from build123d import *

# Parameters (mm, degrees)
BOSS_EXTRUDE1_DEPTH   = 1.6
SKETCH2_R             = 3.45
BOSS_EXTRUDE2_DEPTH   = 1.4
M3X0_5_TAPPED_HOLE1_D = 2.5


with BuildPart() as part:
    # Sketch1 → Boss-Extrude1 (new body)
    with BuildSketch(Plane.XY):
        with BuildLine():
            Line((-6.237396753, 4.481095129), (-3, 5))
            Line((-3, 5), (3, 5))
            Line((3, 5), (6.237396753, 4.481095129))
            ThreePointArc((6.237396753, 4.481095129), (7.141511088, 3.973114811), (7.5, 3))
            Line((7.5, 3), (7.5, -3))
            ThreePointArc((7.5, -3), (7.141511088, -3.973114811), (6.237396753, -4.481095129))
            Line((6.237396753, -4.481095129), (3, -5))
            Line((3, -5), (-3, -5))
            Line((-3, -5), (-6.237396753, -4.481095129))
            ThreePointArc((-6.237396753, -4.481095129), (-7.141511088, -3.973114811), (-7.5, -3))
            Line((-7.5, -3), (-7.5, 3))
            ThreePointArc((-7.5, 3), (-7.141511088, 3.973114811), (-6.237396753, 4.481095129))
        make_face()
    extrude(amount=BOSS_EXTRUDE1_DEPTH)

    # Sketch2 → Boss-Extrude2 (add)
    with BuildSketch(Plane.XY.offset(1.6)):
        Circle(SKETCH2_R)
    extrude(amount=BOSS_EXTRUDE2_DEPTH)

    # M3x0.5 Tapped Hole1 (through all)
    with Locations(Plane.XY.offset(3)):
        with Locations((0, 0)):
            Hole(M3X0_5_TAPPED_HOLE1_D / 2)


solid = part.part
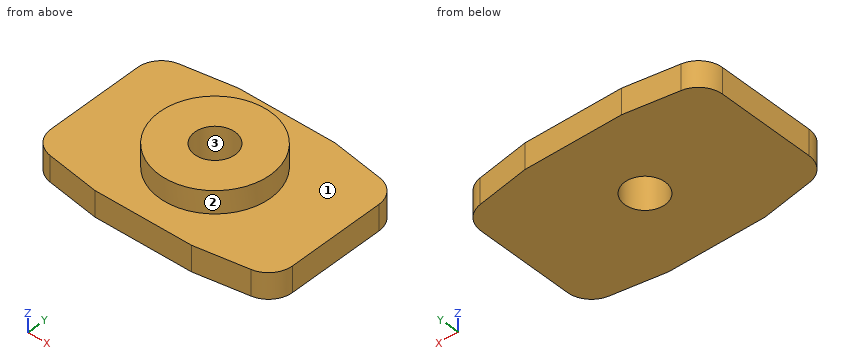
Build history of the part. All positions in model axes, mm. Face numbers are marked on the shaded views. Round coordinates to 2 decimals unless told otherwise and drop trailing zeros. Write each loop counter-clockwise with the first axis right and the second up, starting at its lowest first coordinate (ties: lowest second). Pieces come first, ordered by that corner, then holes. Notation, with made-up numbers: (22.25, -12.75) -> (81.25, -12.75) arc R7 ccw to (81.25, 0.25) -> close; hole circle Ø4 at (44, -11). An arc over 180 degrees is marked (long way). Use one line per item in the form item = value.
Q1. Drill centre lines: L1, parallel to Y at x = 0, z = 2.15; L2, parallel to Y at x = 0, z = 1.45; L3, parallel to Z at x = -3.75, y = -1. Where is each one in solid material? Low to high.
Conclusion:
L1 = -3.45 to -1.25, 1.25 to 3.45
L2 = -5 to -1.25, 1.25 to 5
L3 = 0 to 1.6
Q2. Band-saw the part on D-D, the plane x = -3.25. Write the cut outline in (y, z), then the cut area to 3 significant figures.
Conclusion:
outline = (-4.96, 0) -> (4.96, 0) -> (4.96, 1.6) -> (1.16, 1.6) -> (1.16, 3) -> (-1.16, 3) -> (-1.16, 1.6) -> (-4.96, 1.6) -> close
area = 19.1 mm²
Q3. Band-saw the part on A-A, the plane x = 0. Write the cut outline in (y, z).
Conclusion:
outline = (-5, 0) -> (-1.25, 0) -> (-1.25, 3) -> (-3.45, 3) -> (-3.45, 1.6) -> (-5, 1.6) -> close; (1.25, 0) -> (5, 0) -> (5, 1.6) -> (3.45, 1.6) -> (3.45, 3) -> (1.25, 3) -> close
Q4. Band-saw the part on B-B, the plane y = 0. Write the cut outline in (x, z), then the cut area to 3 significant figures.
Conclusion:
outline = (-7.5, 0) -> (-1.25, 0) -> (-1.25, 3) -> (-3.45, 3) -> (-3.45, 1.6) -> (-7.5, 1.6) -> close; (1.25, 0) -> (7.5, 0) -> (7.5, 1.6) -> (3.45, 1.6) -> (3.45, 3) -> (1.25, 3) -> close
area = 26.2 mm²
Q5. Drop a flat-ended pin along its axis: P1, Ø1.5, axis at x = 0, y = 0, coming from the +Z side. Give the stop position or say it passes through.
Conclusion:
P1 = through
Q6. Band-saw the part on C-C, the plane z = 0.5. Write the cut outline in (x, y), then the cut area to 3 significant figures.
Conclusion:
outline = (-7.5, -3) arc R1.5 ccw to (-6.24, -4.48) -> (-3, -5) -> (3, -5) -> (6.24, -4.48) arc R1.5 ccw to (7.5, -3) -> (7.5, 3) arc R1.5 ccw to (6.24, 4.48) -> (3, 5) -> (-3, 5) -> (-6.24, 4.48) arc R1.5 ccw to (-7.5, 3) -> close; hole circle Ø2.5 at (0, 0)
area = 137 mm²
Q7. Two-plate mould, pull along Y, no slides. Class the marked faces 1, 2 and 3: released by +Y, released by -Y, zero draft, split by the parting line, or undercut.
Conclusion:
face_1 = zero draft
face_2 = split by the parting line
face_3 = undercut
